```python
from build123d import *

# Parameters (mm, degrees)
F0_R      = 20.2
F2_DEPTH  = 25
F1_R      = 20
F3_DEPTH  = 12.5
F3_FACE_R = 20
F4_DEPTH  = 25
F5_R      = 4.181686
F6_DEPTH  = 40
F6_FACE_R = 4.181686
F7_DEPTH  = 25


with BuildPart() as f2:
    # F0 (on Top) → F2 (new body)
    with BuildSketch(Plane.XY):
        Circle(F0_R)
    extrude(amount=F2_DEPTH)

    # F1 (on Top) → F3 (cut, symmetric)
    with BuildSketch(Plane.XY):
        Circle(F1_R)
    extrude(amount=F3_DEPTH, both=True, mode=Mode.SUBTRACT)

    # F3_face (on face) → F4 (cut)
    with BuildSketch(Plane(origin=(0, 0, 12.5), x_dir=(1, 0, 0), z_dir=(0, 0, -1))):
        Circle(F3_FACE_R)
    extrude(amount=-F4_DEPTH, mode=Mode.SUBTRACT)

    # F5 (on Front) → F6 (join)
    with BuildSketch(Plane.XZ):
        with Locations((10.451388, 0)):
            Circle(F5_R)
    extrude(amount=F6_DEPTH)

    # F6_face (on face) → F7 (join)
    with BuildSketch(Plane(origin=(10.451388, 0, 0), x_dir=(1, 0, 0), z_dir=(0, 1, 0))):
        Circle(F6_FACE_R)
    extrude(amount=F7_DEPTH)


solid = f2.part
```
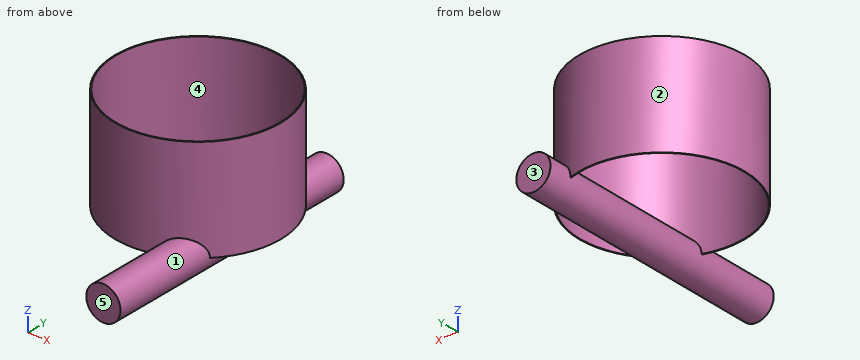
Check sheet for the modelled part. Datum: model origin and axes. Units: mm. Face numbers are marked on the shaded views. A direction names the side the tool comes from. Round coordinates to 2 decimals unless told otherwise and drop trailing zeros. Loops run counter-clockwise (first coordinate to the right, second up) from the corner with the lowest first, then second, coordinate; pieces in that order, holes last. Notation, with made-up numbers: (1, 12) -> (23, 12) arc R19 cw to (23, 33) -> close; hole circle Ø10 at (6, -5). An arc over 180 degrees is marked (long way). Answer in a Markdown table with one row per item.
Q1. Sectioned sample at A-A on y = 0. Enter the section's corners in (x, z), then the cut area to 3 significant figures.
Data:
| item | result |
|---|---|
| outline | (-20.2, 0) -> (-20, 0) -> (-20, 25) -> (-20.2, 25) -> close; circle Ø8.36 at (10.45, 0); (20, 0) -> (20.2, 0) -> (20.2, 25) -> (20, 25) -> close |
| area | 64.9 mm^2 |
Q2. Set-up check for the marked faces 1 and 2: record each of +Z, -Z, +X, -X, +Y, -Y from which the full face is reachable in a straight line by a thin tool's end or side.
Data:
| item | result |
|---|---|
| face 1 | none |
| face 2 | +Z |
Q3. Thickness scan on L1, parallel to Y at x = 0, z = 13.75; L2, parallel to Y at x = 9, z = 10; L3, parallel to X at y = 5, z = 12.5. Record the ranges inside material, lowest first.
Data:
| item | result |
|---|---|
| L1 | y = -20.2 to -20, 20 to 20.2 |
| L2 | y = -18.08 to -17.86, 17.86 to 18.08 |
| L3 | x = -19.57 to -19.36, 19.36 to 19.57 |
Q4. Sectioned sample at C-C on z = 8. Enter the section's corners in (x, y), then the cut area to 3 significant figures.
Data:
| item | result |
|---|---|
| outline | circle Ø40.4 at (0, 0); hole circle Ø40 at (0, 0) |
| area | 25.3 mm^2 |
Q5. Sectioned sample at B-B on x = 0. Enter the section's corners in (y, z), then the cut area to 4 significant figures.
Data:
| item | result |
|---|---|
| outline | (-20.2, 0) -> (-20, 0) -> (-20, 25) -> (-20.2, 25) -> close; (20, 0) -> (20.2, 0) -> (20.2, 25) -> (20, 25) -> close |
| area | 10.00 mm^2 |
Q6. Go/stop test with flat-tipped pins: P1, Ø4, axis at x = 13.5, y = 4.5, coming from the +Z side; P2, Ø10, axis at x = -7.5, y = -9.5, coming from the -Z side; P3, Ø10, axis at x = -10.5, z = 7.5, coming from the +Y side; P4, Ø3, axis at y = -20, z = 0.5, coming from the -X side. Record where each tip stops, or that it passes through.
Data:
| item | result |
|---|---|
| P1 | stops at z = 4.05 |
| P2 | passes through |
| P3 | stops at y = 19.44 |
| P4 | stops at x = -8.11 |
Q7. Sectioned sample at D-D on x = -10. Enter the section's corners in (y, z), then the cut area to 3 significant figures.
Data:
| item | result |
|---|---|
| outline | (-17.55, 0) -> (-17.32, 0) -> (-17.32, 25) -> (-17.55, 25) -> close; (17.32, 0) -> (17.55, 0) -> (17.55, 25) -> (17.32, 25) -> close |
| area | 11.5 mm^2 |
Q8. Release check for a two-part mould opening along Y. For the marked faces 3, 4 and 5 record: released by +Y, released by -Y, zero draft, split by the parting line, or undercut.
Data:
| item | result |
|---|---|
| face 3 | released by +Y |
| face 4 | undercut |
| face 5 | released by -Y |
